Check sheet for the drawn part. Datum: minimum x, y, z corner. Units: mm. Round coordinates to 2 decimals unless told otherwise and drop trailing zeros. Write each loop counter-clockwise with the first axis right and the second up, starting at its lowest first coordinate (ties: lowest second). Pieces come first, ordered by that corner, then holes. Notation, with made-up numbers: (6, 28) - (13, 28) arc R20 cw to (13, 59) - close; hole circle Ø1 at (-40, 83.5). An arc over 180 degrees is marked (long way). Answer as a JSON object with one key per item and string values.
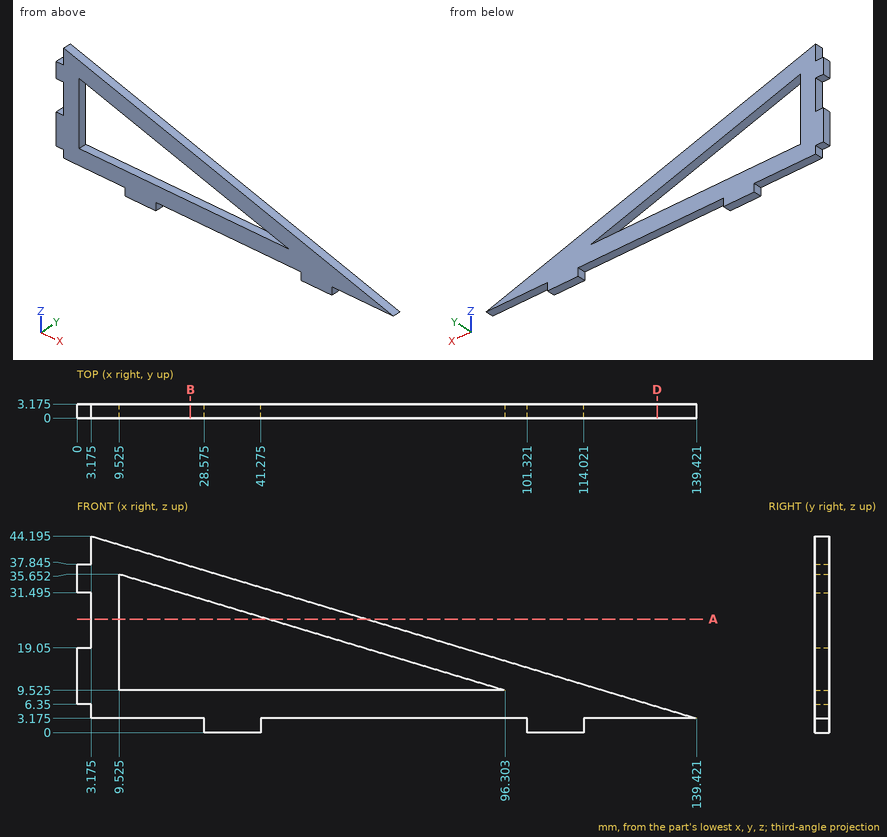
Q1. Section check B-B, the plane x = 25.5. Record the cut outline in (y, z) (1 decimal), then the cut area to 3 significant figures.
Geometry check:
{"outline": "(0, 3.2) - (3.2, 3.2) - (3.2, 9.5) - (0, 9.5) - close; (0, 30.8) - (3.2, 30.8) - (3.2, 37.5) - (0, 37.5) - close", "area": "41.2 mm2"}
Q2. Gauge pin test, flat ends, axial feed: P1, Ø1, axis at y = 1.5, z = 42.5, coming from the -X side (3 decimals); P2, Ø1, axis at x = 57.5, z = 20.5, coming from the +Y side; P3, Ø1, axis at x = 1.5, y = 1, coming from the -Z side; P4, Ø1, axis at y = 2, z = 1.5, coming from the -X side (3 decimals). Record the tip position at first contact, or that the pin passes through.
Geometry check:
{"P1": "stops at x = 3.175", "P2": "passes through", "P3": "stops at z = 6.35", "P4": "stops at x = 28.575"}
Q3. Material ranges on line 1 along Z through (x, y) = (30.5, 1.15) (1 decimal); line 2 along Z through (x, y) = (86.5, 2.7) (1 decimal); line 3 along Z through (x, y) = (111, 0.6), recorded low to high. Write a range as [from, to].
Geometry check:
{"line 1": "z = [0, 9.5], [29.3, 36]", "line 2": "z = [3.2, 9.5], [12.5, 19.1]", "line 3": "z = [0, 11.73]"}
Q4. Section check D-D, the plane x = 130.5. Record the cut outline in (y, z) (1 decimal).
Geometry check:
{"outline": "(0, 3.2) - (3.2, 3.2) - (3.2, 5.9) - (0, 5.9) - close"}
Q5. Section check A-A, the plane z = 25.5. Record the cut outline in (x, y) (1 decimal).
Geometry check:
{"outline": "(3.2, 0) - (9.5, 0) - (9.5, 3.2) - (3.2, 3.2) - close; (43.2, 0) - (65.3, 0) - (65.3, 3.2) - (43.2, 3.2) - close"}
